Source: three-view drawing plus pictorial views. Frame: mm from the lowest corner of the part. A direction names the side the tool comes from. Give positions to 0.01 mm unless a question says otherwise; leave off trailing zeros. Loops run counter-clockwise (first coordinate to the right, second up) from the corner with the lowest first, then second, coordinate; pieces in that order, holes last.
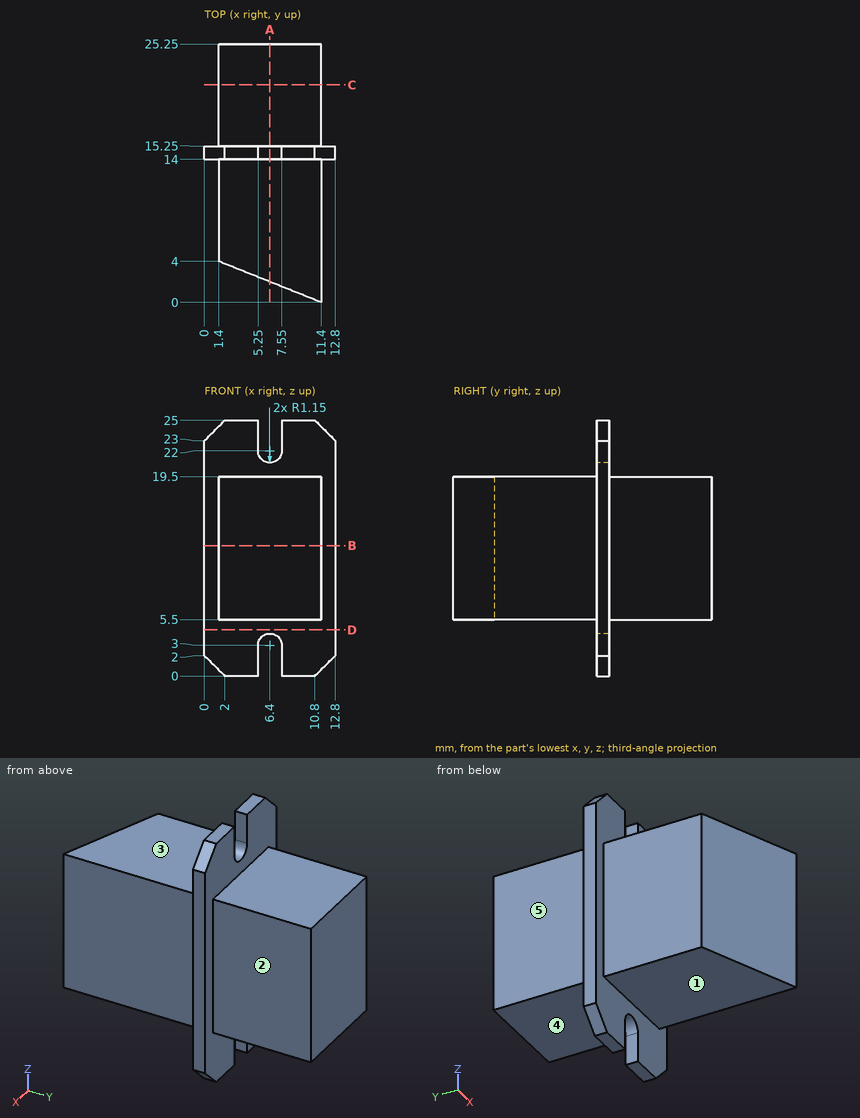
Q1. Material intervals for probe 1 along Y at (x, z) = (1.25, 14); probe 2 along Z at (x, y) = (10, 6.25); probe 3 along X at (y, z) = (7.75, 14), sorted ascending.
Q2. Section query A-A, the plane x = 6.4. Return loops of the section in (y, z).
Q3. Pin query (flat end, axial travel): pin 1 Ø5 at (x, y) = (4, 19) entering from +Z; pin 2 Ø6 at (y, z) = (8, 4.5) entering from -X; pin 3 Ø3 at (x, y) = (6.5, 22) entering from -Z. Return the tip coordinate at first contact, or that it passes through.
Q4. Section query C-C, the plane y = 21.25. Return loops of the section in (x, z).
Q5. Section query B-B, the plane z = 12.75. Return loops of the section in (x, y).
Q6. Reachability of the marked faces 1, 2, 3, 4 and 5 from +Z, -Z, +X, -X, +Y, -Y: full face, straight path, thin tool, end or side. Return the list, or none.
Q7. Section query D-D, the plane z = 4.5. Return loops of the section in (x, y), and give its area (3 significant figures).
Resolved:
1. probe 1: y = 14 to 15.25
1. probe 2: z = 5.5 to 19.5
1. probe 3: x = 1.4 to 11.4
2. outline: (2, 5.5) - (14, 5.5) - (14, 4.15) - (15.25, 4.15) - (15.25, 5.5) - (25.25, 5.5) - (25.25, 19.5) - (15.25, 19.5) - (15.25, 20.85) - (14, 20.85) - (14, 19.5) - (2, 19.5) - close
3. pin 1: stops at z = 19.5
3. pin 2: stops at x = 1.4
3. pin 3: stops at z = 5.5
4. outline: (1.4, 5.5) - (11.4, 5.5) - (11.4, 19.5) - (1.4, 19.5) - close
5. outline: (0, 14) - (1.4, 14) - (1.4, 4) - (11.4, 0) - (11.4, 14) - (12.8, 14) - (12.8, 15.25) - (11.4, 15.25) - (11.4, 25.25) - (1.4, 25.25) - (1.4, 15.25) - (0, 15.25) - close
6. face 1: -Z, +X, -X, -Y
6. face 2: +Z, -Z, +X, +Y
6. face 3: +Z, +X, -X, -Y
6. face 4: -Z, +X, -X, +Y
6. face 5: +Z, -Z, -X, +Y
7. outline: (0, 14) - (12.8, 14) - (12.8, 15.25) - (0, 15.25) - close
7. area: 16.0 mm2
